Geometry check sheet. Reference: the model listing, model coordinates, mm. Round coordinates to 2 decimals unless told otherwise and drop trailing zeros. Order: outer loops, then holes, each group sorted by start corner. A loop starts at its lowest first (then second) coordinate and runs counter-clockwise, first axis right, second up. Notation, with made-up numbers: (6.25, 88.25) - (21.25, 88.25) arc R17 cw to (21.25, 92.25) - close; hole circle Ø7 at (40, -14.75). An arc over 180 degrees is marked (long way). Answer as CSV lines item,"result". Start each with the question number.
Solid Edge part; units mm, degrees
sketch "Sketch1" plane through (0, 85, 0) normal (0, -1, 0) x (1, 0, 0)
  line L0 (-135.3603, -10) -> (-129.3548, -26.5)
  line L1 (-129.3548, -26.5) -> (-99.4453, -26.5)
  line L2 (-99.4453, -26.5) -> (-89.8001, 0)
  line L3 (-139, 0) -> (-89.8001, 0)
  line L4 (-139, 0) -> (-135.3603, -10)
  circle A0 centre (-123.1516, -17.3415) radius 2.45
  circle A1 centre (-131.5, -5) radius 2.45
  circle A2 centre (-108.8981, -13) radius 7.95
extrude "Extrusionsausprägung_1" add sketch "Sketch1" along normal blind 18
properties material "(None)"
1. Section check A-A on x = -131.5. Record the boundary of the cut face in (y, z).
2. Draft check along X on faces 1 (the face through (-94.69, 76.13, -13.44)), 2 (the face through (-125.6, 76.1, -17.4)), 3 (the face through (-115, 76, 0)). Enter one of: released by +X, released by -X, zero draft, split by the parting line, or undercut.
3. Go/stop test with flat-tipped pins: pin 1 Ø1.5 at (y, z) = (76, -7.5) entering from -X; pin 2 Ø6 at (y, z) = (78.5, -13.5) entering from +X; pin 3 Ø1.5 at (x, z) = (-104.5, -8) entering from -Y; pin 4 Ø3 at (y, z) = (77.5, -5.5) entering from -X. Record where each tip stops, or that it passes through.
4. Section check D-D on z = -6. Record the boundary of the cut face in (x, y).
5. Section check C-C on y = 80.25. Record the boundary of the cut face in (x, z), plus the area to 3 significant figures.
6. Thickness scan on probe 1 along Z at (x, y) = (-111, 76); probe 2 along X at (y, z) = (78.75, -6.5); probe 3 along Z at (x, y) = (-105, 72.75). Record the ranges inside material, lowest first.
7. Section check B-B on z = -14. Record the boundary of the cut face in (x, y).
Numbers:
1,outline,"(67, -20.61) - (85, -20.61) - (85, -7.45) - (67, -7.45) - close; (67, -2.55) - (85, -2.55) - (85, 0) - (67, 0) - close"
2,face 1,"released by +X"
2,face 2,"undercut"
2,face 3,"zero draft"
3,pin 1,"stops at x = -136.54"
3,pin 2,"stops at x = -93.62"
3,pin 3,"passes through"
3,pin 4,"stops at x = -137.54"
4,outline,"(-136.82, 67) - (-133.74, 67) - (-133.74, 85) - (-136.82, 85) - close; (-129.26, 67) - (-112.67, 67) - (-112.67, 85) - (-129.26, 85) - close; (-105.13, 67) - (-91.98, 67) - (-91.98, 85) - (-105.13, 85) - close"
5,outline,"(-139, 0) - (-135.36, -10) - (-129.35, -26.5) - (-99.45, -26.5) - (-89.8, 0) - close; hole circle Ø4.9 at (-131.5, -5); hole circle Ø4.9 at (-123.15, -17.34); hole circle Ø15.9 at (-108.9, -13)"
5,area,"812 mm2"
6,probe 1,"z = -26.5 to -20.67, -5.33 to 0"
6,probe 2,"x = -136.63 to -133.44, -129.56 to -113.48, -104.32 to -92.17"
6,probe 3,"z = -26.5 to -19.93, -6.07 to 0"
7,outline,"(-133.9, 67) - (-116.78, 67) - (-116.78, 85) - (-133.9, 85) - close; (-101.01, 67) - (-94.9, 67) - (-94.9, 85) - (-101.01, 85) - close"
